Here's how the part is built. I have some questions about the finished solid (model axes, mm). A direction names the side the tool comes from. Round coordinates to 2 decimals unless told otherwise and drop trailing zeros. Loops run counter-clockwise (first coordinate to the right, second up) from the corner with the lowest first, then second, coordinate; pieces in that order, holes last. Notation, with made-up numbers: (86, 80) - (122, 80) arc R24 cw to (122, 115) - close; hole circle Ø1 at (19.25, 8.5). An arc over 180 degrees is marked (long way). Answer as a JSON object with one key per item and string values. Group by question number.
1) I want a section at D-D, the plane x = -29.5. Please give me the cut outline in (y, z).
2) If we mould it in two halves opening along Z, with no side actions, what happens to faces 4 (the face through (-28, -75.3, -49)), 5 (the face through (-46.203, -80.19, -33.029)), 6 (the face through (-25.541, -34.103, -49.105))? For each: pulls with the +Z half, pulls with the -Z half, needs draft (parallel to the pull), parting line crosses it, or undercut.
3) Will these pins go through, and if not, where does the flat tip stop? P1, Ø2, axis at y = -75.5, z = -35, coming from the +X side; P2, Ø1, axis at x = -44, y = -24.5, coming from the +Z side; P3, Ø6, axis at y = -29, z = -15, coming from the -X side.
4) I want a section at B-B, the plane z = 15. Please give me the cut outline in (x, y).
5) I want a section at C-C, the plane y = -80.3. Please give me the cut outline in (x, z).
6) Which directions (+Z, -Z, +X, -X, +Y, -Y) give clear straight access to the entire face, cutting with the end or side of a thin tool? Please do faces 1 (the face through (-5.502, -80.19, 56.527)), 2 (the face through (5.502, -80.19, -56.527)), 3 (the face through (51.7, -80.2, -23.5)).
7) I want a section at A-A, the plane x = 0. Please give me the cut outline in (y, z).
8) If I drill on line 1 along X through (y, z) = (-45, 0); line 2 along Z through (x, y) = (-16, -64.5), over which ranges is the centre line in solid material (lowest first)? Write a range as [from, to].
Autodesk Inventor part; units mm, degrees
ref_plane "YZ Plane" through (0, 0, 0) normal (1, 0, 0) x (0, 1, 0)
ref_plane "XZ Plane" through (0, 0, 0) normal (0, 1, 0) x (-1, 0, 0)
ref_plane "XY Plane" through (0, 0, 0) normal (0, 0, 1) x (1, 0, 0)
sketch "Esquisse1" plane through (0, 0, 0) normal (0, 1, 0) x (-1, 0, 0)
  line L0 (0, -80.29) -> (0, 80.29) construction
  line L1 (-80.29, 0) -> (80.29, 0) construction
  circle A0 centre (0, 0) radius 57.35
  circle A1 centre (0, 0) radius 55.35
  circle A2 centre (0, 0) radius 16 construction
  circle A3 centre (0, 0) radius 57.35 construction
  dimension "d0" = 2
extrude "Extrusion1" add sketch "Esquisse1" against normal blind 89.3
sketch "Esquisse2" plane through (0, 0, 0) normal (1, 0, 0) x (0, 1, 0)
  line L0 (-80.3, 18.5) -> (-80.3, -18.5) construction
  line L1 (-85.3, 18.5) -> (-85.3, -18.5)
  line L2 (-75.3, -18.5) -> (-75.3, 18.5)
  arc A0 (-75.3, 18.5) -> (-85.3, 18.5) centre (-80.3, 18.5) ccw
  arc A1 (-85.3, -18.5) -> (-75.3, -18.5) centre (-80.3, -18.5) ccw
  line L3 (-89.3, 57.35) -> (-89.3, -57.35) construction
  line L4 (-81.6, 0) -> (13.6, 0) construction
  point P0 (0, 0)
  point P1 (-80.3, 0)
  dimension "d3" = 4
  dimension "d4" = 5
  dimension "d5" = 37
extrude "Extrusion2" cut sketch "Esquisse2" against normal blind 68
pattern_circular "Réseau circulaire1" count 6 over 360 about axis through (0, -10, 0) along (0, 1, 0) of "Extrusion2"
properties part number "Colossus_7kW_Rotor_body"
Outcome:
{
 "1": {"outline": "(-89.3, -49.18) - (-85.3, -49.18) - (-85.3, -46.83) - (-89.3, -46.83) - close; (-89.3, 46.83) - (-85.3, 46.83) - (-85.3, 49.18) - (-89.3, 49.18) - close; (-75.3, -49.18) - (0, -49.18) - (0, -46.83) - (-75.3, -46.83) - close; (-75.3, 46.83) - (0, 46.83) - (0, 49.18) - (-75.3, 49.18) - close"},
 "2": {"face 4": "needs draft", "face 5": "pulls with the -Z half", "face 6": "undercut"},
 "3": {"P1": "x = 46.18", "P2": "z = 37.37", "P3": "x = -56.08"},
 "4": {"outline": "(-55.35, -89.3) - (-53.28, -89.3) - (-53.28, -85.3) - (-55.35, -85.3) - close; (-55.35, -75.3) - (-53.28, -75.3) - (-53.28, 0) - (-55.35, 0) - close; (53.28, -89.3) - (55.35, -89.3) - (55.35, -85.3) - (53.28, -85.3) - close; (53.28, -75.3) - (55.35, -75.3) - (55.35, 0) - (53.28, 0) - close"},
 "5": {"outline": "(-52.31, -23.5) arc R57.35 ccw to (-46.51, -33.56) - (-45.41, -31.65) arc R55.35 cw to (-50.11, -23.5) - close; (-52.31, 23.5) - (-50.11, 23.5) arc R55.35 cw to (-45.41, 31.65) - (-46.51, 33.56) arc R57.35 ccw to start; (-5.81, -57.06) arc R57.35 ccw to (5.81, -57.06) - (4.71, -55.15) arc R55.35 cw to (-4.71, -55.15) - close; (-5.81, 57.06) - (-4.71, 55.15) arc R55.35 cw to (4.71, 55.15) - (5.81, 57.06) arc R57.35 ccw to start; (45.41, -31.65) - (46.51, -33.56) arc R57.35 ccw to (52.31, -23.5) - (50.11, -23.5) arc R55.35 cw to start; (45.41, 31.65) arc R55.35 cw to (50.11, 23.5) - (52.31, 23.5) arc R57.35 ccw to (46.51, 33.56) - close"},
 "6": {"face 1": "-X", "face 2": "+X", "face 3": "+X, -X"},
 "7": {"outline": "(-89.3, -57.35) - (0, -57.35) - (0, -55.35) - (-89.3, -55.35) - close; (-89.3, 55.35) - (0, 55.35) - (0, 57.35) - (-89.3, 57.35) - close"},
 "8": {"line 1": "[-57.35, -55.35], [55.35, 57.35]", "line 2": "[-55.07, -52.99], [52.99, 55.07]"}
}
